Verification items for the finished model (mm, model axes). A direction names the side the tool comes from. Coordinates: 2 decimals unless noted, no trailing zeros. Loops run counter-clockwise (first coordinate to the right, second up) from the corner with the lowest first, then second, coordinate; pieces in that order, holes last. Notation, with made-up numbers: (-32.5, 26.5) - (-6.5, 26.5) arc R21 ccw to (-6.5, 57.5) - close; hole circle Ø2 at (36, 18). An arc over 180 degrees is marked (long way). One line per item, written item: value. Start each with the question number.
(1) Section check D-D (x = -14). Record the boundary of the cut face in (y, z).
(2) Gauge pin test, flat ends, axial feed: P1, Ø1.5, axis at y = 2, z = 4.5, coming from the -X side; P2, Ø14, axis at x = 0, y = 0, coming from the -Z side; P3, Ø4, axis at x = -11, z = 4, coming from the -Y side. Record the tip position at first contact, or that the pin passes through.
(3) Section check A-A (x = 0). Record the boundary of the cut face in (y, z).
(4) Draft check along Y on faces 1 (the face through (12.845, 11.692, 4.93)), 2 (the face through (12.853, -11.672, 4.93)), 3 (the face through (-9, 0, 0)), 4 (the face through (-0.1, 10.5, 5.1)). Enter one of: +Y half, -Y half, draft (parallel to the pull), parting line (faces both ways), or undercut.
(5) Thickness scan on probe 1 along Y at (x, z) = (0, 3.5); probe 2 along Y at (x, z) = (0, 8.85); probe 3 along X at (y, z) = (-14.5, 5). Record the ranges inside material, lowest first. Write a range as [from, to].
(6) Section check C-C (x = 4). Record the boundary of the cut face in (y, z), plus the area to 3 significant figures.
(7) Section check B-B (y = 0). Record the boundary of the cut face in (x, z), plus the area to 3 significant figures.
(8) Set-up check for faces 5 (the face through (-6, 4, 10)), 6 (the face through (4, -5, 7)): record each of +Z, -Z, +X, -X, +Y, -Y from which the full face is reachable in a straight line by a thin tool's end or side.
Autodesk Inventor part; units mm, degrees
ref_plane "YZ Plane" through (0, 0, 0) normal (1, 0, 0) x (0, 1, 0)
ref_plane "XZ Plane" through (0, 0, 0) normal (0, 1, 0) x (-1, 0, 0)
ref_plane "XY Plane" through (0, 0, 0) normal (0, 0, 1) x (1, 0, 0)
sketch "Sketch1" plane through (0, 0, 0) normal (0, 0, 1) x (1, 0, 0)
  circle A0 centre (0, 0) radius 6
  circle A1 centre (0, 0) radius 17.5
  dimension "d0" = 12
  dimension "d1" = 35
extrude "Extrusion1" add sketch "Sketch1" along normal blind 10
sketch "Sketch4" plane through (0, 0, 0) normal (0, 0, -1) x (-1, 0, 0)
  circle A0 centre (0, 0) radius 13 construction
  point P0 (0, -13)
  point P1 (0, 13)
  dimension "d7" = 26
hole "Hole1" at (0, -13, 0) at (0, 13, 0) direction (0, 0, 1) diameter 5 end through all
sketch "Sketch5" plane through (0, 0, 0) normal (0, 0, -1) x (-1, 0, 0)
  circle A0 centre (0, 0) radius 8.15
  dimension "d15" = 16.3
extrude "Extrusion3" cut sketch "Sketch5" against normal blind 7
sketch "Sketch6" plane through (0, 0, 10) normal (0, 0, 1) x (1, 0, 0)
  line L0 (13, -11.7154) -> (13, 11.7154)
  circle A0 centre (0, 0) radius 17.5
  circle A1 centre (0, -13) radius 2.5 construction
  circle A2 centre (0, 13) radius 2.5 construction
  line L1 (0, -13) -> (0, 13) construction
  dimension "d22" = 13
extrude "Extrusion4" cut sketch "Sketch6" against normal through all contours L0 A0 picked at (13.8164, -2.7401)
fillet "Fillet2" radius 2 2 edges at (13, -11.7154, 5) (13, 11.7154, 5)
properties part number "0008-10-034 Suport_Rulment" material "ABS Plastic"
Responses:
1. outline: (-10.5, 0) - (10.5, 0) - (10.5, 10) - (-10.5, 10) - close
2. P1: stops at x = -17.46
2. P2: stops at z = 7
2. P3: stops at y = -15.01
3. outline: (-17.5, 0) - (-15.5, 0) - (-15.5, 10) - (-17.5, 10) - close; (-10.5, 0) - (-8.15, 0) - (-8.15, 7) - (-6, 7) - (-6, 10) - (-10.5, 10) - close; (6, 7) - (8.15, 7) - (8.15, 0) - (10.5, 0) - (10.5, 10) - (6, 10) - close; (15.5, 0) - (17.5, 0) - (17.5, 10) - (15.5, 10) - close
4. face 1: +Y half
4. face 2: -Y half
4. face 3: draft
4. face 4: undercut
5. probe 1: y = [-17.5, -15.5], [-10.5, -8.15], [8.15, 10.5], [15.5, 17.5]
5. probe 2: y = [-17.5, -15.5], [-10.5, -6], [6, 10.5], [15.5, 17.5]
5. probe 3: x = [-9.8, -2], [2, 9.8]
6. outline: (-17.04, 0) - (-7.1, 0) - (-7.1, 7) - (-4.47, 7) - (-4.47, 10) - (-17.04, 10) - close; (4.47, 7) - (7.1, 7) - (7.1, 0) - (17.04, 0) - (17.04, 10) - (4.47, 10) - close
6. area: 214 mm²
7. outline: (-17.5, 0) - (-8.15, 0) - (-8.15, 7) - (-6, 7) - (-6, 10) - (-17.5, 10) - close; (6, 7) - (8.15, 7) - (8.15, 0) - (13, 0) - (13, 10) - (6, 10) - close
7. area: 155 mm²
8. face 5: +Z, +X, -X, +Y, -Y
8. face 6: -Z
